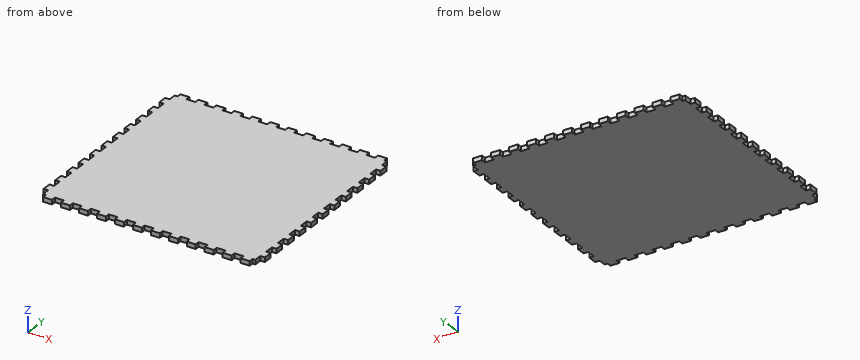
```python
from build123d import *

# Parameters (mm, degrees)
BOSS_EXTRUDE1_DEPTH = 5.715


with BuildPart() as part:
    # Model → Boss-Extrude1 (new body)
    with BuildSketch(Plane.XY):
        Polygon((584.688856535, 28.575245224), (588.246340911, 28.575245224), (588.246340911, 22.860238699), (599.673519312, 22.860238699), (599.673519312, 28.575245224), (611.104241025, 28.575245224), (611.104241025, 22.860238699), (622.534962737, 22.860238699), (622.534962737, 28.575245224), (633.965684449, 28.575245224), (633.965684449, 22.860238699), (645.396406161, 22.860238699), (645.396406161, 28.575245224), (656.823584562, 28.575245224), (656.823584562, 22.860238699), (668.254306275, 22.860238699), (668.254306275, 28.575245224), (679.685027987, 28.575245224), (679.685027987, 22.860238699), (691.115749699, 22.860238699), (691.115749699, 28.575245224), (702.546471411, 28.575245224), (702.546471411, 22.860238699), (713.973649812, 22.860238699), (713.973649812, 28.575245224), (725.404371525, 28.575245224), (725.404371525, 22.860238699), (736.835093237, 22.860238699), (736.835093237, 28.575245224), (748.265814949, 28.575245224), (748.265814949, 22.860238699), (759.696536661, 22.860238699), (759.696536661, 28.575245224), (771.123715063, 28.575245224), (771.123715063, 22.860238699), (782.554436775, 22.860238699), (782.554436775, 28.575245224), (793.985158487, 28.575245224), (793.985158487, 22.860238699), (805.415880199, 22.860238699), (805.415880199, 28.575245224), (816.846601911, 28.575245224), (816.846601911, 22.860238699), (828.273780313, 22.860238699), (828.273780313, 28.575245224), (839.704502025, 28.575245224), (839.704502025, 22.860238699), (851.135223737, 22.860238699), (851.135223737, 28.575245224), (854.689164803, 28.575245224), (854.689164803, 38.560083395), (860.404525659, 38.560083395), (860.404525659, 49.990096445), (854.689164803, 49.990096445), (854.689164803, 61.420109495), (860.404525659, 61.420109495), (860.404525659, 72.850122545), (854.689164803, 72.850122545), (854.689164803, 84.280135595), (860.404525659, 84.280135595), (860.404525659, 95.710148645), (854.689164803, 95.710148645), (854.689164803, 107.140161695), (860.404525659, 107.140161695), (860.404525659, 118.570174745), (854.689164803, 118.570174745), (854.689164803, 130.000187795), (860.404525659, 130.000187795), (860.404525659, 141.430200846), (854.689164803, 141.430200846), (854.689164803, 152.860213896), (860.404525659, 152.860213896), (860.404525659, 164.290226946), (854.689164803, 164.290226946), (854.689164803, 175.720239996), (860.404525659, 175.720239996), (860.404525659, 187.150253046), (854.689164803, 187.150253046), (854.689164803, 198.580266096), (860.404525659, 198.580266096), (860.404525659, 210.010279146), (854.689164803, 210.010279146), (854.689164803, 221.440292196), (860.404525659, 221.440292196), (860.404525659, 232.870305246), (854.689164803, 232.870305246), (854.689164803, 244.300318296), (860.404525659, 244.300318296), (860.404525659, 255.730331346), (854.689164803, 255.730331346), (854.689164803, 267.160344396), (860.404525659, 267.160344396), (860.404525659, 278.590357446), (854.689164803, 278.590357446), (854.689164803, 288.575408216), (851.135223737, 288.575408216), (851.135223737, 294.290414741), (839.704502025, 294.290414741), (839.704502025, 288.575408216), (828.273780313, 288.575408216), (828.273780313, 294.290414741), (816.846601911, 294.290414741), (816.846601911, 288.575408216), (805.415880199, 288.575408216), (805.415880199, 294.290414741), (793.985158487, 294.290414741), (793.985158487, 288.575408216), (782.554436775, 288.575408216), (782.554436775, 294.290414741), (771.123715063, 294.290414741), (771.123715063, 288.575408216), (759.696536661, 288.575408216), (759.696536661, 294.290414741), (748.265814949, 294.290414741), (748.265814949, 288.575408216), (736.835093237, 288.575408216), (736.835093237, 294.290414741), (725.404371525, 294.290414741), (725.404371525, 288.575408216), (713.973649812, 288.575408216), (713.973649812, 294.290414741), (702.546471411, 294.290414741), (702.546471411, 288.575408216), (691.115749699, 288.575408216), (691.115749699, 294.290414741), (679.685027987, 294.290414741), (679.685027987, 288.575408216), (668.254306275, 288.575408216), (668.254306275, 294.290414741), (656.823584562, 294.290414741), (656.823584562, 288.575408216), (645.396406161, 288.575408216), (645.396406161, 294.290414741), (633.965684449, 294.290414741), (633.965684449, 288.575408216), (622.534962737, 288.575408216), (622.534962737, 294.290414741), (611.104241025, 294.290414741), (611.104241025, 288.575408216), (599.673519312, 288.575408216), (599.673519312, 294.290414741), (588.246340911, 294.290414741), (588.246340911, 288.575408216), (584.688856535, 288.575408216), (584.688856535, 278.590357446), (578.973495678, 278.590357446), (578.973495678, 267.160344396), (584.688856535, 267.160344396), (584.688856535, 255.730331346), (578.973495678, 255.730331346), (578.973495678, 244.300318296), (584.688856535, 244.300318296), (584.688856535, 232.870305246), (578.973495678, 232.870305246), (578.973495678, 221.440292196), (584.688856535, 221.440292196), (584.688856535, 210.010279146), (578.973495678, 210.010279146), (578.973495678, 198.580266096), (584.688856535, 198.580266096), (584.688856535, 187.150253046), (578.973495678, 187.150253046), (578.973495678, 175.720239996), (584.688856535, 175.720239996), (584.688856535, 164.290226946), (578.973495678, 164.290226946), (578.973495678, 152.860213896), (584.688856535, 152.860213896), (584.688856535, 141.430200846), (578.973495678, 141.430200846), (578.973495678, 130.000187795), (584.688856535, 130.000187795), (584.688856535, 118.570174745), (578.973495678, 118.570174745), (578.973495678, 107.140161695), (584.688856535, 107.140161695), (584.688856535, 95.710148645), (578.973495678, 95.710148645), (578.973495678, 84.280135595), (584.688856535, 84.280135595), (584.688856535, 72.850122545), (578.973495678, 72.850122545), (578.973495678, 61.420109495), (584.688856535, 61.420109495), (584.688856535, 49.990096445), (578.973495678, 49.990096445), (578.973495678, 38.560083395), (584.688856535, 38.560083395), align=None)
    extrude(amount=BOSS_EXTRUDE1_DEPTH)


solid = part.part
```
CAD build for the part. Positions are in the model's coordinates, mm. Coordinates: 2 decimals unless noted, no trailing zeros. Order: outer loops, then holes, each group sorted by start corner. A loop starts at its lowest first (then second) coordinate and runs counter-clockwise, first axis right, second up. Notation, with made-up numbers: (27.5, 35.25) -> (42.5, 35.25) arc R20 cw to (42.5, 55.25) -> close; hole circle Ø10 at (80.5, 9.5). An arc over 180 degrees is marked (long way). Use one line per item in the form item = value. Start each with the question number.
1) Drill centre lines: L1, parallel to X at y = 146, z = 1.8; L2, parallel to Y at x = 695, z = 0.9. Where is each one in solid material? Low to high. Write a range as [from, to].
2) Drop flat-ended pins along their axis: pin 1 (1.7 mm diameter, centred on y = 291.5, z = 4, fed in from -X); pin 2 (3 mm diameter, centred on y = 291.5, z = 3.5, fed in from +X); pin 3 (3 mm diameter, centred on x = 582.5, z = 2.5, fed in from -Y). Give the stop position or say it passes through.
3) Band-saw the part on A-A on y = 191.5. Give the cut face in (x, z) (3 decimals), then the cut area to 3 significant figures.
Entries:
q1.L1 = [584.69, 854.69]
q1.L2 = [28.58, 288.58]
q2.pin_1 = 588.25
q2.pin_2 = 851.14
q2.pin_3 = 38.56
q3.outline = (584.689, 0) -> (854.689, 0) -> (854.689, 5.715) -> (584.689, 5.715) -> close
q3.area = 1,540 mm2
